from build123d import *

# Parameters (mm, degrees)
F1_DEPTH  = 40
F2_W      = 25
F2_H      = 25
F3_DEPTH  = 80
F4_W      = 225
F4_H      = 25
F5_DEPTH  = 25
F7_DEPTH  = 40
F9_DEPTH  = 40
F10_R     = 6
F11_DEPTH = 400.001
F12_W     = 40
F12_H     = 40
F12_W_2   = 38
F12_H_2   = 38
F13_DEPTH = 40
F14_W     = 40
F14_H     = 40
F14_W_2   = 38
F14_H_2   = 38
F15_DEPTH = 40
F16_R     = 4
F17_DEPTH = 25
F18_R     = 4
F19_DEPTH = 25
F21_DEPTH = 40
F23_DEPTH = 40


with BuildPart() as f1:
    # F0 (on Top) → F1 (new body)
    with BuildSketch(Plane.XY):
        Polygon((0, 650), (0, 0), (40, 0), (40, 610), (360, 610), (360, 0), (400, 0), (400, 650), align=None)
    extrude(amount=F1_DEPTH)

    # F2 (on face) → F3 (join)
    with BuildSketch(Plane(origin=(0, 650, 0), x_dir=(-1, 0, 0), z_dir=(0, 1, 0))):
        with Locations((-100, 25)):
            Rectangle(F2_W, F2_H)
        with Locations((-300, 25)):
            Rectangle(F2_W, F2_H)
    extrude(amount=F3_DEPTH)

    # F4 (on face) → F5 (join)
    with BuildSketch(Plane(origin=(0, 730, 0), x_dir=(-1, 0, 0), z_dir=(0, 1, 0))):
        with Locations((-200, 25)):
            Rectangle(F4_W, F4_H)
    extrude(amount=F5_DEPTH)

    # F6 (on face) → F7 (join)
    with BuildSketch(Plane(origin=(0, 0, 0), x_dir=(0, -1, 0), z_dir=(-1, 0, 0))):
        Polygon((-40, 40), (0, 40), (-52.8980942125, 340), (-92.8980942125, 340), align=None)
    extrude(amount=-F7_DEPTH)

    # F8 (on face) → F9 (join)
    with BuildSketch(Plane.YZ.offset(400)):
        Polygon((52.8980942125, 340), (0, 40), (40, 40), (92.8980942125, 340), align=None)
    extrude(amount=-F9_DEPTH)

    # F10 (on face) → F11 (cut, through all)
    with BuildSketch(Plane.YZ.offset(400)):
        with Locations((20, 20)):
            Circle(F10_R)
    extrude(amount=-F11_DEPTH, mode=Mode.SUBTRACT)

    # F12 (on face) → F13 (join)
    with BuildSketch(Plane.YZ.offset(400)):
        with Locations((72.8980942125, 360)):
            Rectangle(F12_W, F12_H)
        with Locations((72.8980942125, 360)):
            Rectangle(F12_W_2, F12_H_2, mode=Mode.SUBTRACT)
    extrude(amount=-F13_DEPTH)

    # F14 (on face) → F15 (join)
    with BuildSketch(Plane(origin=(0, 0, 0), x_dir=(0, -1, 0), z_dir=(-1, 0, 0))):
        with Locations((-72.8980942125, 360)):
            Rectangle(F14_W, F14_H)
        with Locations((-72.8980942125, 360)):
            Rectangle(F14_W_2, F14_H_2, mode=Mode.SUBTRACT)
    extrude(amount=-F15_DEPTH)

    # F16 (on face) → F17 (cut)
    with BuildSketch(Plane.XY.offset(380)):
        with Locations((20, 72.8980942125)):
            Circle(F16_R)
    extrude(amount=-F17_DEPTH, mode=Mode.SUBTRACT)

    # F18 (on face) → F19 (cut)
    with BuildSketch(Plane.XY.offset(380)):
        with Locations((380, 72.8980942125)):
            Circle(F18_R)
    extrude(amount=-F19_DEPTH, mode=Mode.SUBTRACT)

    # F20 (on face) → F21 (join)
    with BuildSketch(Plane.YZ.offset(400)):
        Polygon((75.0933335322, 239.0241844507), (190, 40), (236.1880215352, 40), (85.8992778316, 300.3077399002), align=None)
    extrude(amount=-F21_DEPTH)

    # F22 (on face) → F23 (join)
    with BuildSketch(Plane(origin=(0, 0, 0), x_dir=(0, -1, 0), z_dir=(-1, 0, 0))):
        Polygon((-236.1880215352, 40), (-190, 40), (-75.0933335322, 239.0241844507), (-85.8992778316, 300.3077399002), align=None)
    extrude(amount=-F23_DEPTH)


solid = f1.part
Verification items for the finished model (mm, model axes). A direction names the side the tool comes from. Round coordinates to 2 decimals unless told otherwise and drop trailing zeros. Loops run counter-clockwise (first coordinate to the right, second up) from the corner with the lowest first, then second, coordinate; pieces in that order, holes last. Notation, with made-up numbers: (13.5, 62) - (26.5, 62) arc R10 ccw to (26.5, 79) - close; hole circle Ø10 at (-10.5, 1). An arc over 180 degrees is marked (long way). Write item = value, one per line.
Q1. Sectioned sample at D-D on y = 178.5. Record the boundary of the cut face in (x, z), plus the area to 3 significant figures.
Here are the results:
outline = (0, 0) - (40, 0) - (40, 40) - (0, 40) - close; (0, 59.92) - (40, 59.92) - (40, 139.92) - (0, 139.92) - close; (360, 0) - (400, 0) - (400, 40) - (360, 40) - close; (360, 59.92) - (400, 59.92) - (400, 139.92) - (360, 139.92) - close
area = 9,600 mm^2
Q2. Material ranges on L1, parallel to X at y = 225, z = 22; L2, parallel to Y at x = 20, z = 379.45; L3, parallel to Z at x = 377, y = 136.5, recorded low to high.
Here are the results:
L1 = 0 to 40, 360 to 400
L2 = 52.9 to 68.9, 76.9 to 92.9
L3 = 0 to 40, 132.66 to 212.66
Q3. Sectioned sample at A-A on x = 272. Record the boundary of the cut face in (y, z), plus the area to 4 significant figures.
Here are the results:
outline = (610, 0) - (650, 0) - (650, 40) - (610, 40) - close; (730, 12.5) - (755, 12.5) - (755, 37.5) - (730, 37.5) - close
area = 2,225 mm^2
Q4. Depth check by flat-ended pin: pin 1 (12 mm diameter, centred on x = 384.5, z = 361, fed in from +Y); pin 2 (20 mm diameter, centred on x = 378.5, z = 354.5, fed in from -Y); pin 3 (20 mm diameter, centred on x = 216.5, z = 29, fed in from -Y). Enter the tip coordinate at first touch or a pass-through.
Here are the results:
pin_1 = 92.9
pin_2 = 52.9
pin_3 = 610
Q5. Mould release check, pull along X, two halves, no side actions. Record for faces 1 (the flat face through (20, 92.898, 360)), 2 (the flat face through (0, 206, 64)), 3 (the flat face through (360, 191, 92)): +X half, -X half, draft (parallel to the pull), parting line (faces both ways), or undercut.
Here are the results:
face_1 = draft
face_2 = -X half
face_3 = undercut
Q6. Tool access check on faces 4 (the flat face through (201, 730, 25)), 5 (the flat face through (198, 610, 20)), 6 (the flat face through (202, 737, 37.5)), 7 (the flat face through (380, 73, 341)). Record the directions out of +Z, -Z, +X, -X, +Y, -Y that give a thin tool (end or side, any length) a straight path to the whole face; none if there is none.
Here are the results:
face_4 = +Z, -Z
face_5 = +Z, -Z, -Y
face_6 = +Z, +X, -X, +Y
face_7 = +X, -X
Q7. Sectioned sample at B-B on y = 697. Record the boundary of the cut face in (x, z), plus the area to 3 significant figures.
Here are the results:
outline = (87.5, 12.5) - (112.5, 12.5) - (112.5, 37.5) - (87.5, 37.5) - close; (287.5, 12.5) - (312.5, 12.5) - (312.5, 37.5) - (287.5, 37.5) - close
area = 1,250 mm^2
Q8. Sectioned sample at C-C on z = 112.5. Record the boundary of the cut face in (x, y).
Here are the results:
outline = (0, 12.78) - (40, 12.78) - (40, 52.78) - (0, 52.78) - close; (0, 148.14) - (40, 148.14) - (40, 194.33) - (0, 194.33) - close; (360, 12.78) - (400, 12.78) - (400, 52.78) - (360, 52.78) - close; (360, 148.14) - (400, 148.14) - (400, 194.33) - (360, 194.33) - close
